Can you work these out from the model? Positions are in its coordinate system, mm. Round coordinates to 2 decimals unless told otherwise and drop trailing zeros. Order: outer loops, then holes, each group sorted by start corner. A loop starts at its lowest first (then second) coordinate and runs counter-clockwise, first axis right, second up.
Q1. If we section it at C-C (z = 12): Please give me the cut outline in (x, y).
Q2. Will these pins go through, and if not, where does the flat tip stop? P1, Ø8, axis at x = -52.5, z = 7, coming from the +Y side; P2, Ø1.5, axis at y = 47, z = 11.5, coming from the +X side; P3, Ø3, axis at x = -53, z = 11, coming from the -Y side; P4, Ø1, axis at y = 36.5, z = 15.5, coming from the -X side.
Q3. If we section it at B-B (x = -53.5): Please give me the cut outline in (y, z), plus the area to 3 significant figures.
Q4. If I drill on line 1 (Y direction, x = -52.75, z = 14.75); line 2 (X direction, y = 45, z = 10.75); line 3 (Y direction, x = -56.75, z = 8.5), over which ranges is the centre line in solid material (lowest first)?
Q5. If we section it at A-A (y = 35.5): Please give me the cut outline in (x, z), plus the area to 3 significant figures.
from build123d import *

# Parameters (mm, degrees)
SKETCH1_W             = 128.922622712
SKETCH1_H             = 108.547542538
SKETCH1_W_2           = 124.922622712
SKETCH1_H_2           = 104.547542538
BOSS_EXTRUDE1_DEPTH   = 50
SKETCH2_R             = 48.496570744
BOSS_EXTRUDE2_DEPTH   = 50
SKETCH3_R             = 6.994110628
BOSS_EXTRUDE3_DEPTH   = 20
SKETCH3_R_2           = 6.120691225
BOSS_EXTRUDE3_2_DEPTH = 20


with BuildPart() as part:
    # Sketch1 → Boss-Extrude1 (new body)
    with BuildSketch(Plane.XY):
        Rectangle(SKETCH1_W, SKETCH1_H)
        Rectangle(SKETCH1_W_2, SKETCH1_H_2, mode=Mode.SUBTRACT)
    extrude(amount=BOSS_EXTRUDE1_DEPTH)


with BuildPart() as body_2:
    # Sketch2 → Boss-Extrude2 (new body)
    with BuildSketch(Plane.XY):
        with Locations(Location((0, 0, 0), (0, 0, 180))):
            Circle(SKETCH2_R)
    extrude(amount=BOSS_EXTRUDE2_DEPTH)


with BuildPart() as body_3:
    # Sketch3 → Boss-Extrude3 (new body)
    with BuildSketch(Plane.XY):
        with Locations((-51.126362865, 41.516845757)):
            Circle(SKETCH3_R)
    extrude(amount=BOSS_EXTRUDE3_DEPTH)


with BuildPart() as body_4:
    # Sketch3 → Boss-Extrude3 2 (new body)
    with BuildSketch(Plane.XY):
        with Locations((46.461548735, 43.755956539)):
            Circle(SKETCH3_R_2)
    extrude(amount=BOSS_EXTRUDE3_2_DEPTH)


solid = body_3.part
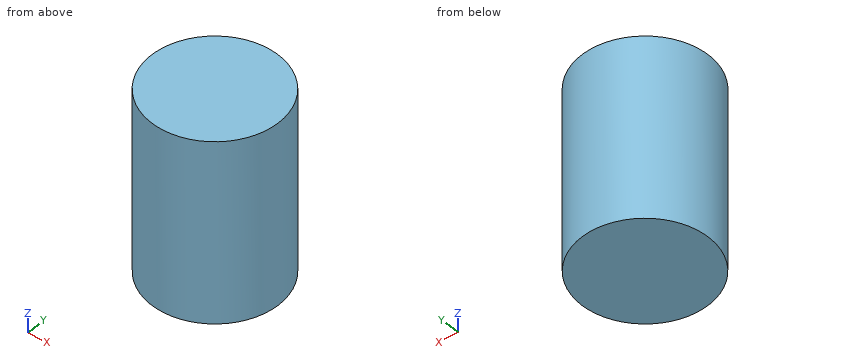
Solution:
1. outline: circle Ø13.99 at (-51.13, 41.52)
2. P1: stops at y = 48.51
2. P2: stops at x = -45.98
2. P3: stops at y = 34.53
2. P4: stops at x = -56.47
3. outline: (34.94, 0) - (48.1, 0) - (48.1, 20) - (34.94, 20) - close
3. area: 263 mm2
4. line 1: y = 34.71 to 48.32
4. line 2: x = -57.19 to -45.06
4. line 3: y = 37.36 to 45.68
5. outline: (-54.69, 0) - (-47.56, 0) - (-47.56, 20) - (-54.69, 20) - close
5. area: 143 mm2
